Part model, mm, in its own coordinate system. Coordinates: 2 decimals unless noted, no trailing zeros. Write each loop counter-clockwise with the first axis right and the second up, starting at its lowest first coordinate (ties: lowest second). Pieces come first, ordered by that corner, then holes. Notation, with made-up numbers: (42.5, 19.25) - (95.5, 19.25) arc R20 cw to (95.5, 47.25) - close; hole circle Ø7 at (-3, 4). An arc over 180 degrees is marked (long way). Write each question's results on one line, items separated by ' | '.
from build123d import *

# Parameters (mm, degrees)
SKETCH1_R           = 2.5
SKETCH1_R_2         = 1.500000002
BOSS_EXTRUDE1_DEPTH = 3


with BuildPart() as part:
    # Sketch1 → Boss-Extrude1 (new body)
    with BuildSketch(Plane.XY):
        with BuildLine():
            Line((-36.744474703, 67.343539136), (27.095525297, 67.958794059))
            ThreePointArc((27.095525297, 67.958794059), (45.803097829, 63.138855192), (27.191895339, 57.959258429))
            Line((27.191895339, 57.959258429), (-36.648104661, 57.344003506))
            Line((-36.648104661, 57.344003506), (-36.744474703, 67.343539136))
        make_face()
        with Locations((35.803562199, 63.04248515)):
            Circle(SKETCH1_R, mode=Mode.SUBTRACT)
        with Locations((10.804723125, 62.801560043)):
            Circle(SKETCH1_R_2, mode=Mode.SUBTRACT)
    extrude(amount=BOSS_EXTRUDE1_DEPTH)


solid = part.part
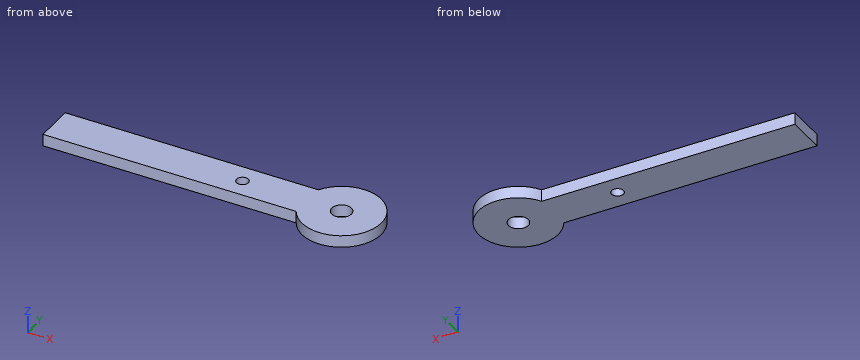
(1) Saw through at D-D on y = 54.5. Write the cut outline in (x, z), then the cut area to 3 significant figures.
Return value:
outline: (30.6, 0) - (41, 0) - (41, 3) - (30.6, 3) - close | area: 31.2 mm^2
(2) Saw through at A-A on y = 62. Write the cut outline in (x, z).
Return value:
outline: (-36.69, 0) - (9.54, 0) - (9.54, 3) - (-36.69, 3) - close; (12.07, 0) - (33.53, 0) - (33.53, 3) - (12.07, 3) - close; (38.08, 0) - (45.75, 0) - (45.75, 3) - (38.08, 3) - close
(3) Saw through at B-B on z = 0.8. Write the cut outline in (x, y), then the cut area to 3 significant figures.
Return value:
outline: (-36.74, 67.34) - (-36.65, 57.34) - (27.19, 57.96) arc R10 ccw (long way) to (27.1, 67.96) - close; hole circle Ø3 at (10.8, 62.8); hole circle Ø5 at (35.8, 63.04) | area: 917 mm^2
(4) Flat gauge pins, fed straight in: P1, Ø1, axis at x = -3.5, y = 57, coming from the +Z side; P2, Ø5, axis at x = 10.8, y = 62.8, coming from the +Z side. Where does each tip first touch, or does it go through?
Return value:
P1: passes through | P2: stops at z = 3
(5) Saw through at C-C on x = 40.5. Write the cut outline in (y, z), then the cut area to 3 significant figures.
Return value:
outline: (54.21, 0) - (71.87, 0) - (71.87, 3) - (54.21, 3) - close | area: 53.0 mm^2
(6) Wall check: line 1 (Y direction, x = 36, z = 0.5); line 2 (X direction, y = 62.25, z = 2.75); line 3 (X direction, y = 62, z = 0.45). Give the ranges that are in metal, low to high. Write a range as from..to.
Return value:
line 1: y = 53.04..60.55, 65.53..73.04 | line 2: x = -36.7..9.41, 12.2..33.43, 38.17..45.77 | line 3: x = -36.69..9.54, 12.07..33.53, 38.08..45.75
